Can you work these out from the model? Positions are in its coordinate system, mm. Face numbers are marked on the shaded views. A direction names the side the tool comes from. Round coordinates to 2 decimals unless told otherwise and drop trailing zeros. Loops run counter-clockwise (first coordinate to the right, second up) from the corner with the lowest first, then second, coordinate; pieces in that order, holes last.
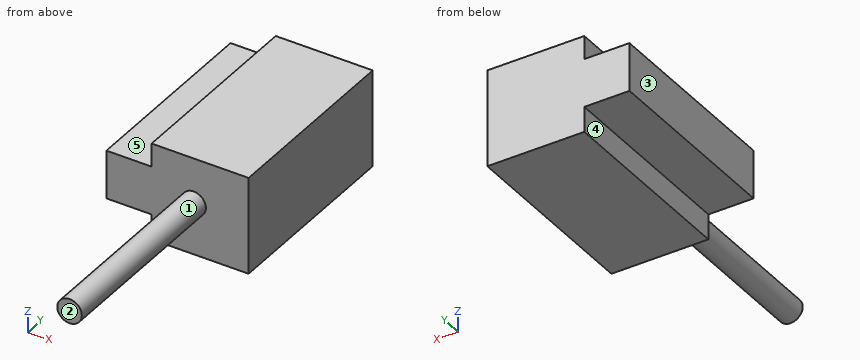
```python
from build123d import *

# Parameters (mm, degrees)
F0_W     = 118.379154
F0_H     = 126.638353
F1_DEPTH = 508
F2_R     = 32.145306
F3_DEPTH = 508
F4_DEPTH = 508
F5_DEPTH = 508


with BuildPart() as f1:
    # F0 (on Front) → F1 (new body)
    with BuildSketch(Plane.XZ):
        Polygon((-254, 0), (0, 0), (0, 254), (-254, 254), (-254, 192.787692), (-254, 66.149339), align=None)
        with Locations((-313.189577, 129.468515)):
            Rectangle(F0_W, F0_H)
    extrude(amount=F1_DEPTH)

    # F2 (on face) → F3 (join)
    with BuildSketch(Plane.XZ.offset(508)):
        with Locations((-143.956617, 134.362638)):
            Circle(F2_R)
    extrude(amount=-F3_DEPTH)

    # F2 (on face) + F1_face (on face) → F4 (join)
    with BuildSketch(Plane.XZ.offset(508)):
        with Locations((-143.956617, 134.362638)):
            Circle(F2_R)
    with BuildSketch(Plane(origin=(-162.106588, -508, 127.465446), x_dir=(1, 0, 0), z_dir=(0, -1, 0))):
        Polygon((-91.893412, -127.465446), (162.106588, -127.465446), (162.106588, 126.534554), (-91.893412, 126.534554), (-91.893412, 65.322246), (-210.272566, 65.322246), (-210.272566, -61.316107), (-91.893412, -61.316107), align=None)
    extrude(amount=-F4_DEPTH)

    # F2 (on face) → F5 (join)
    with BuildSketch(Plane.XZ.offset(508)):
        with Locations((-143.956617, 134.362638)):
            Circle(F2_R)
    extrude(amount=F5_DEPTH)


solid = f1.part
```
(1) If I drill on line 1 (X direction, y = -466, z = 62.5); line 2 (Y direction, x = -19, z = 222.5), over which ranges is the centre line in solid material (lowest first)?
(2) For pin 1 (1.5 mm diameter, centred on x = -311, z = 142.5, fed in from -Y); pin 2 (8 mm diameter, centred on x = -264.5, z = 121.5, fed in from +Y); pin 3 (1 mm diameter, centred on y = -157, z = 56, fed in from -X), each with a flat end and sliding along its axis, tell me the tip position at first contact or that it passes through.
(3) Which directions (+Z, -Z, +X, -X, +Y, -Y) give clear straight access to the entire face, cutting with the end or side of a thin tool? Please do the marked faces 1, 2, 3, 4 and 5.
(4) Suppose I cut it at B-B (x = -291.5). Write out the boundary of the cut face in (y, z).
(5) Suppose I cut it at C-C (z = 148.5). Write out the boundary of the cut face in (x, y), then the cut area to 4 significant figures.
(6) Suppose I cut it at A-A (y = -111). Write out the boundary of the cut face in (x, z), then the cut area to 3 significant figures.
(7) Suppose I cut it at D-D (z = 238). Write out the boundary of the cut face in (x, y), then the cut area to 3 significant figures.
Check result:
1. line 1: x = -254 to 0
1. line 2: y = -508 to 0
2. pin 1: stops at y = -508
2. pin 2: stops at y = 0
2. pin 3: stops at x = -254
3. face 1: -Y
3. face 2: +Z, -Z, +X, -X, -Y
3. face 3: +Z, -Z, -X, +Y, -Y
3. face 4: -Z, -X, +Y, -Y
3. face 5: +Z, -X, +Y, -Y
4. outline: (-508, 66.15) - (0, 66.15) - (0, 192.79) - (-508, 192.79) - close
5. outline: (-372.38, -508) - (-172.83, -508) - (-172.83, -1016) - (-115.09, -1016) - (-115.09, -508) - (0, -508) - (0, 0) - (-372.38, 0) - close
5. area: 218,500 mm2
6. outline: (-372.38, 66.15) - (-254, 66.15) - (-254, 0) - (0, 0) - (0, 254) - (-254, 254) - (-254, 192.79) - (-372.38, 192.79) - close
6. area: 79,500 mm2
7. outline: (-254, -508) - (0, -508) - (0, 0) - (-254, 0) - close
7. area: 129,000 mm2
